from build123d import *

# Parameters (mm, degrees)
SKETCH_W     = 34.25
SKETCH_H     = 72
PAD_DEPTH    = 2
SKETCH001_W  = 3.9
SKETCH001_H  = 69.8
PAD001_DEPTH = 3


with BuildPart() as part:
    # Sketch → Pad (new body)
    with BuildSketch(Plane.XY):
        Rectangle(SKETCH_W, SKETCH_H)
    extrude(amount=PAD_DEPTH)

    # Sketch001 → Pad001 (join)
    with BuildSketch(Plane.XY):
        with Locations((-14.125, 0)):
            Rectangle(SKETCH001_W, SKETCH001_H)
    extrude(amount=-PAD001_DEPTH)


solid = part.part
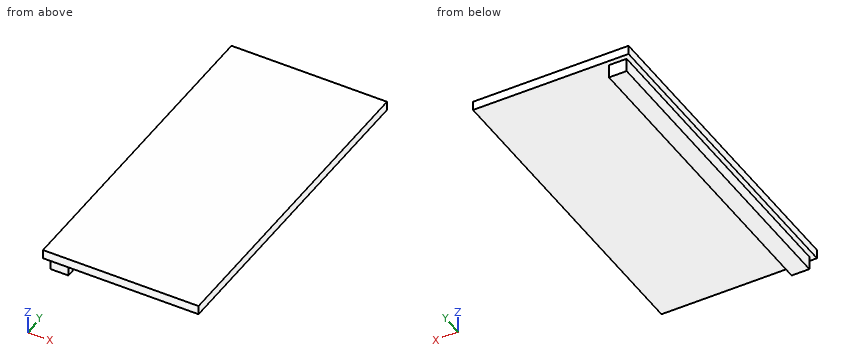
Verification items for the finished model (mm, model axes). Coordinates: 2 decimals unless noted, no trailing zeros. Order: outer loops, then holes, each group sorted by start corner. A loop starts at its lowest first (then second) coordinate and runs counter-clockwise, first axis right, second up. Notation, with made-up numbers: M -23,-0.75 L 27,-0.75 A16 cw 27,30.25 Z; hole C 2,9 d10. An arc over 180 degrees is marked long. One line per item, written item: value. Start each with the question number.
Item 1: Sectioned sample at C-C on z = -1.8. Record the cut outline in (x, y) (3 decimals).
Item 2: Sectioned sample at A-A on y = 15.5. Record the cut outline in (x, z) (3 decimals), then the cut area to 3 significant figures.
Item 3: Depth check by flat-ended pin: P1, Ø4, axis at x = -4, y = 25.5, coming from the -Z side; P2, Ø17, axis at x = -8, y = -15.5, coming from the -Z side; P3, Ø0.9, axis at x = -13.5, z = -1.5, coming from the +Y side; P4, Ø0.9, axis at x = -14.5, z = -2, coming from the -Y side. Enter the tip coordinate at first touch or a pass-through.
Item 4: Thickness scan on probe 1 along Z at (x, y) = (9, -22); probe 2 along X at (y, z) = (6, -2.1) (3 decimals); probe 3 along Y at (x, z) = (-15, -0.4). Record the ranges inside material, lowest first.
Item 5: Sectioned sample at B-B on x = -13. Record the cut outline in (y, z).
Item 6: Sectioned sample at D-D on x = -4. Record the cut outline in (y, z).
Calculated:
1. outline: M -16.075,-34.9 L -12.175,-34.9 L -12.175,34.9 L -16.075,34.9 Z
2. outline: M -17.125,0 L -16.075,0 L -16.075,-3 L -12.175,-3 L -12.175,0 L 17.125,0 L 17.125,2 L -17.125,2 Z
2. area: 80.2 mm^2
3. P1: z = 0
3. P2: z = -3
3. P3: y = 34.9
3. P4: y = -34.9
4. probe 1: 0 to 2
4. probe 2: -16.075 to -12.175
4. probe 3: -34.9 to 34.9
5. outline: M -36,0 L -34.9,0 L -34.9,-3 L 34.9,-3 L 34.9,0 L 36,0 L 36,2 L -36,2 Z
6. outline: M -36,0 L 36,0 L 36,2 L -36,2 Z
